For this review, take the finished solid that the model builds, in its own axes (mm). A direction names the side the tool comes from. Give positions to 0.01 mm unless a question says otherwise; leave off trailing zeros. Write each loop counter-clockwise with the first axis right and the second up, starting at its lowest first coordinate (ties: lowest second). Pieces come first, ordered by that corner, then holes. Notation, with made-up numbers: M -16,77.25 L 35,77.25 A22 ccw 35,104.25 Z; hole C 2.5,36.25 d7. An arc over 180 degrees is marked long. One line per item, written item: value. Start each with the question number.
Item 1: Consider section C-C, the plane z = 9.5. Write out the cut boundary in (x, y).
Item 2: Clearance check with flat-ended pins moving along their axes: pin 1 Ø4 at (x, z) = (11.5, -10.5) entering from +Y; pin 2 Ø1 at (x, z) = (-13, -1.5) entering from -Y; pin 3 Ø2 at (y, z) = (1.5, -8.5) entering from +X; pin 4 Ø8 at (y, z) = (4, 16.5) entering from +X. State where each tip first meets the part, or that it passes through.
Item 3: Consider section A-A, the plane x = 10.5. Write out the cut boundary in (y, z), and give its area (3 significant figures).
Item 4: Consider section B-B, the plane z = -3. Write out the cut boundary in (x, y).
Item 5: Consider section D-D, the plane x = 23. Write out the cut boundary in (y, z).
Item 6: To check wall thickness, follow probe 1 along Z at (x, y) = (-3, 1.5); probe 2 along X at (y, z) = (10.75, -2); probe 3 along Z at (x, y) = (-5, 11). State the ranges of each line that lie inside material, in increasing order.
Item 7: Mouldability with a two-part tool opening along Y and no side actions: class faces 1 (the face through (-15.5, 3, 25.7)), 2 (the face through (-4, 1, -1.328)) as released by +Y, released by -Y, zero draft, split by the parting line, or undercut.
Item 8: Tool access review of faces 3 (the face through (12, 1, -7.475)), 4 (the face through (21, 14, -4.468)), 5 (the face through (-13, 5, 2.366)), 6 (the face through (26, 13, 27)): name each direction out of +Z, -Z, +X, -X, +Y, -Y from which nothing blocks a thin tool from reaching the whole face with its end or side.
```python
from build123d import *

# Parameters (mm, degrees)
SKETCH1_W               = 36
SKETCH1_H               = 49
BOSS_EXTRUDE1_DEPTH     = 2
SKETCH2_W               = 36
SKETCH2_H               = 49
SKETCH2_W_2             = 32
SKETCH2_H_2             = 45
BOSS_EXTRUDE2_DEPTH     = 13
CUT_EXTRUDE1_DEPTH      = 5
CUT_EXTRUDE1_DEPTH_BACK = 48.529259103
SKETCH3_W               = 7.5
SKETCH3_H               = 2
SKETCH4_W               = 4.670437484
SKETCH4_H               = 3.853110924
CUT_EXTRUDE2_DEPTH      = 41.051989913
SKETCH10_W              = 2
SKETCH10_H              = 19
CUT_EXTRUDE6_DEPTH      = 3
SKETCH11_W              = 8
SKETCH11_H              = 7
CUT_EXTRUDE7_DEPTH      = 2
SKETCH12_W              = 5
SKETCH12_H              = 3
BOSS_EXTRUDE3_DEPTH     = 5
SKETCH13_W              = 5
SKETCH13_H              = 3
BOSS_EXTRUDE4_DEPTH     = 5
SKETCH14_R              = 0.775
CUT_EXTRUDE8_DEPTH      = 44.046736753
SKETCH15_R              = 1.275
CUT_EXTRUDE9_DEPTH      = 1
CUT_EXTRUDE10_START     = -1
SKETCH16_R              = 1.275
CUT_EXTRUDE10_DEPTH     = 1
FILLET2_R               = 10
SKETCH17_W              = 2
SKETCH17_H              = 4
CUT_EXTRUDE11_DEPTH     = 59.103279375
SKETCH18_W              = 2
SKETCH18_H              = 4
CUT_EXTRUDE12_DEPTH     = 53.763912582
SKETCH19_W              = 37.08283529
SKETCH19_H              = 2
CUT_EXTRUDE13_DEPTH     = 2
SKETCH20_W              = 37.08283529
SKETCH20_H              = 2
BOSS_EXTRUDE5_DEPTH     = 2
SKETCH21_W              = 2
SKETCH21_H              = 28
CUT_EXTRUDE14_DEPTH     = 2
SKETCH22_W              = 2
SKETCH22_H              = 28
BOSS_EXTRUDE6_DEPTH     = 2
SKETCH23_W              = 2
SKETCH23_H              = 34.1
CUT_EXTRUDE16_DEPTH     = 1.5
SKETCH24_W              = 2
SKETCH24_H              = 34.1
BOSS_EXTRUDE7_DEPTH     = 1.5


with BuildPart() as part:
    # Sketch1 → Boss-Extrude1 (new body)
    with BuildSketch(Plane(origin=(0, 0, 0), x_dir=(1, 0, 0), z_dir=(0, 1, 0))):
        with Locations((4.385964912, -5.131578947)):
            Rectangle(SKETCH1_W, SKETCH1_H)
    extrude(amount=BOSS_EXTRUDE1_DEPTH)

    # Sketch2 → Boss-Extrude2 (add)
    with BuildSketch(Plane(origin=(0, 2, 0), x_dir=(1, 0, 0), z_dir=(0, 1, 0))):
        with Locations((4.385964912, -5.131578947)):
            Rectangle(SKETCH2_W, SKETCH2_H)
        with Locations((4.385964912, -5.131578947)):
            Rectangle(SKETCH2_W_2, SKETCH2_H_2, mode=Mode.SUBTRACT)
    extrude(amount=BOSS_EXTRUDE2_DEPTH)

    # Sketch3 → Cut-Extrude1 (cut, two sides: drawn at the far end of the back side and taken through both)
    with BuildSketch(Plane.ZY.offset(-20.385964912).offset(-CUT_EXTRUDE1_DEPTH_BACK)):
        with Locations((-8.218421053, 14)):
            Rectangle(SKETCH3_W, SKETCH3_H)
    extrude(amount=CUT_EXTRUDE1_DEPTH + CUT_EXTRUDE1_DEPTH_BACK, mode=Mode.SUBTRACT)

    # Sketch4 → Cut-Extrude2 (cut, through all)
    with BuildSketch(Plane.XZ):
        with Locations((11.852478182, 20.598290589)):
            Rectangle(SKETCH4_W, SKETCH4_H)
        with Locations((-4.147521818, 20.598290589)):
            Rectangle(SKETCH4_W, SKETCH4_H)
        with Locations((11.852478182, 10.598290589)):
            Rectangle(SKETCH4_W, SKETCH4_H)
        with Locations((11.852478182, 0.598290589)):
            Rectangle(SKETCH4_W, SKETCH4_H)
        with Locations((11.852478182, -9.401709411)):
            Rectangle(SKETCH4_W, SKETCH4_H)
        with Locations((-4.147521818, 10.598290589)):
            Rectangle(SKETCH4_W, SKETCH4_H)
        with Locations((-4.147521818, 0.598290589)):
            Rectangle(SKETCH4_W, SKETCH4_H)
        with Locations((-4.147521818, -9.401709411)):
            Rectangle(SKETCH4_W, SKETCH4_H)
    extrude(amount=-CUT_EXTRUDE2_DEPTH, mode=Mode.SUBTRACT)

    # Sketch10 → Cut-Extrude6 (cut)
    with BuildSketch(Plane(origin=(0, 15, 0), x_dir=(1, 0, 0), z_dir=(0, 1, 0))):
        with Locations((-12.614035088, 7.868421053)):
            Rectangle(SKETCH10_W, SKETCH10_H)
    extrude(amount=-CUT_EXTRUDE6_DEPTH, mode=Mode.SUBTRACT)

    # Sketch11 → Cut-Extrude7 (cut)
    with BuildSketch(Plane.ZY.offset(13.614035088)):
        with Locations((-1.634350226, 5.5)):
            Rectangle(SKETCH11_W, SKETCH11_H)
    extrude(amount=-CUT_EXTRUDE7_DEPTH, mode=Mode.SUBTRACT)

    # Sketch12 → Boss-Extrude3 (add)
    with BuildSketch(Plane.ZY.offset(13.614035088)):
        with Locations((-16.868421053, 1.5)):
            Rectangle(SKETCH12_W, SKETCH12_H)
        with Locations((27.131578947, 13.5)):
            Rectangle(SKETCH12_W, SKETCH12_H)
        with Locations((27.131578947, 1.5)):
            Rectangle(SKETCH12_W, SKETCH12_H)
    extrude(amount=BOSS_EXTRUDE3_DEPTH)

    # Sketch13 → Boss-Extrude4 (add)
    with BuildSketch(Plane(origin=(22.385964912, 0, 0), x_dir=(0, 0, -1), z_dir=(1, 0, 0))):
        with Locations((16.868421053, 1.5)):
            Rectangle(SKETCH13_W, SKETCH13_H)
        with Locations((-27.131578947, 13.5)):
            Rectangle(SKETCH13_W, SKETCH13_H)
        with Locations((-27.131578947, 1.5)):
            Rectangle(SKETCH13_W, SKETCH13_H)
        with Locations((16.868421053, 13.5)):
            Rectangle(SKETCH13_W, SKETCH13_H)
    extrude(amount=BOSS_EXTRUDE4_DEPTH)

    # Sketch14 → Cut-Extrude8 (cut, through all)
    with BuildSketch(Plane.XZ):
        with Locations(Location((24.885964912, -16.868421053, 0), (0, 0, 270))):
            Circle(SKETCH14_R)
        with Locations(Location((-16.114035088, -16.868421053, 0), (0, 0, 270))):
            Circle(SKETCH14_R)
        with Locations(Location((-16.114035088, 27.131578947, 0), (0, 0, 270))):
            Circle(SKETCH14_R)
        with Locations(Location((24.885964912, 27.131578947, 0), (0, 0, 270))):
            Circle(SKETCH14_R)
    extrude(amount=-CUT_EXTRUDE8_DEPTH, mode=Mode.SUBTRACT)

    # Sketch15 → Cut-Extrude9 (cut)
    with BuildSketch(Plane(origin=(0, 3, 0), x_dir=(1, 0, 0), z_dir=(0, 1, 0))):
        with Locations(Location((24.885964912, 16.868421053, 0), (0, 0, 270))):
            Circle(SKETCH15_R)
        with Locations(Location((24.885964912, -27.131578947, 0), (0, 0, 270))):
            Circle(SKETCH15_R)
        with Locations(Location((-16.114035088, -27.131578947, 0), (0, 0, 270))):
            Circle(SKETCH15_R)
        with Locations(Location((-16.114035088, 16.868421053, 0), (0, 0, 270))):
            Circle(SKETCH15_R)
    extrude(amount=-CUT_EXTRUDE9_DEPTH, mode=Mode.SUBTRACT)

    # Sketch16 → Cut-Extrude10 (cut)
    with BuildSketch(Plane.XZ.offset(-12).offset(CUT_EXTRUDE10_START)):
        with Locations(Location((-16.114035088, 27.131578947, 0), (0, 0, 90))):
            Circle(SKETCH16_R)
        with Locations(Location((24.885964912, 27.131578947, 0), (0, 0, 90))):
            Circle(SKETCH16_R)
        with Locations(Location((24.885964912, -16.868421053, 0), (0, 0, 90))):
            Circle(SKETCH16_R)
    extrude(amount=CUT_EXTRUDE10_DEPTH, mode=Mode.SUBTRACT)

    # Fillet2
    # the kernel refuses this fillet: 10 mm, written as the material it adds along each edge
    with BuildSketch(Plane(origin=(-13.614035088, 0, -14.368421053), x_dir=(0, 0, 1), z_dir=(0, 1, 0)), Plane(origin=(22.385964912, 0, 24.631578947), x_dir=(0, 0, -1), z_dir=(0, 1, 0))) as fillet2_piece_1:
        with BuildLine():
            CenterArc((8.660254038, -10), FILLET2_R, 90, 60)
            Line((0, -5), (0, 0))
            Line((0, 0), (8.660254038, 0))
        make_face()
    extrude(amount=3)
    with BuildSketch(Plane(origin=(22.385964912, 0, -14.368421053), x_dir=(0, 0, 1), z_dir=(0, 1, 0)), Plane(origin=(-13.614035088, 0, 24.631578947), x_dir=(0, 0, -1), z_dir=(0, 1, 0))) as fillet2_piece_2:
        with BuildLine():
            CenterArc((8.660254038, 10), FILLET2_R, 210, 60)
            Line((0, 5), (0, 0))
            Line((0, 0), (8.660254038, 0))
        make_face()
    extrude(amount=3)

    # Sketch17 → Cut-Extrude11 (cut, through all)
    with BuildSketch(Plane.XY.offset(29.631578947)):
        with Locations((-3.340209091, 6.894489406)):
            Rectangle(SKETCH17_W, SKETCH17_H)
        with Locations((5.343190897, 6.894489406)):
            Rectangle(SKETCH17_W, SKETCH17_H)
        with Locations((13.309543319, 6.894489406)):
            Rectangle(SKETCH17_W, SKETCH17_H)
    extrude(amount=-CUT_EXTRUDE11_DEPTH, mode=Mode.SUBTRACT)

    # Sketch18 → Cut-Extrude12 (cut, through all)
    with BuildSketch(Plane.ZY.offset(13.614035088)):
        with Locations((11.893757697, 6.4242408)):
            Rectangle(SKETCH18_W, SKETCH18_H)
        with Locations((19.784308777, 6.4242408)):
            Rectangle(SKETCH18_W, SKETCH18_H)
    extrude(amount=-CUT_EXTRUDE12_DEPTH, mode=Mode.SUBTRACT)

    # Sketch19 → Cut-Extrude13 (cut)
    with BuildSketch(Plane(origin=(0, 15, 0), x_dir=(1, 0, 0), z_dir=(0, 1, 0))):
        with Locations((4.927382557, 18.368421053)):
            Rectangle(SKETCH19_W, SKETCH19_H)
    extrude(amount=-CUT_EXTRUDE13_DEPTH, mode=Mode.SUBTRACT)

    # Sketch20 → Boss-Extrude5 (add)
    with BuildSketch(Plane(origin=(0, 13, 0), x_dir=(1, 0, 0), z_dir=(0, 1, 0))):
        with Locations((4.927382557, 18.368421053)):
            Rectangle(SKETCH20_W, SKETCH20_H)
    extrude(amount=BOSS_EXTRUDE5_DEPTH)

    # Sketch21 → Cut-Extrude14 (cut)
    with BuildSketch(Plane(origin=(0, 15, 0), x_dir=(1, 0, 0), z_dir=(0, 1, 0))):
        with Locations((-12.614035088, -15.631578947)):
            Rectangle(SKETCH21_W, SKETCH21_H)
    extrude(amount=-CUT_EXTRUDE14_DEPTH, mode=Mode.SUBTRACT)

    # Sketch22 → Boss-Extrude6 (add)
    with BuildSketch(Plane(origin=(0, 13, 0), x_dir=(1, 0, 0), z_dir=(0, 1, 0))):
        with Locations((-12.614035088, -15.631578947)):
            Rectangle(SKETCH22_W, SKETCH22_H)
    extrude(amount=BOSS_EXTRUDE6_DEPTH)

    # Sketch23 → Cut-Extrude16 (cut)
    with BuildSketch(Plane(origin=(0, 15, 0), x_dir=(1, 0, 0), z_dir=(0, 1, 0))):
        with Locations((21.385964912, -12.581578947)):
            Rectangle(SKETCH23_W, SKETCH23_H)
    extrude(amount=-CUT_EXTRUDE16_DEPTH, mode=Mode.SUBTRACT)

    # Sketch24 → Boss-Extrude7 (add)
    with BuildSketch(Plane(origin=(0, 13.5, 0), x_dir=(1, 0, 0), z_dir=(0, 1, 0))):
        with Locations((21.385964912, -12.581578947)):
            Rectangle(SKETCH24_W, SKETCH24_H)
    extrude(amount=BOSS_EXTRUDE7_DEPTH)


solid = part.part
```
Model answer:
1. outline: M -13.61,0 L -6.48,0 L -6.48,2 L -11.61,2 L -11.61,15 L -13.61,15 Z; M -1.81,0 L 9.52,0 L 9.52,2 L -1.81,2 Z; M 14.19,0 L 22.39,0 L 22.39,15 L 20.39,15 L 20.39,2 L 14.19,2 Z
2. pin 1: stops at y = 2
2. pin 2: stops at y = 0
2. pin 3: stops at x = 23.13
2. pin 4: stops at x = 23.41
3. outline: M 0,-19.37 L 15,-19.37 L 15,-17.37 L 2,-17.37 L 2,-11.33 L 0,-11.33 Z; M 0,-7.48 L 2,-7.48 L 2,-1.33 L 0,-1.33 Z; M 0,2.52 L 2,2.52 L 2,8.67 L 0,8.67 Z; M 0,12.52 L 2,12.52 L 2,18.67 L 0,18.67 Z; M 0,22.52 L 2,22.52 L 2,27.63 L 15,27.63 L 15,29.63 L 0,29.63 Z
3. area: 119 mm2
4. outline: M -13.61,0 L 22.39,0 L 22.39,15 L 20.39,15 L 20.39,2 L -13.61,2 Z; M -13.61,9 L -11.61,9 L -11.61,12 L -13.61,12 Z
5. outline: M 0,-19.37 L 3,-19.37 L 3,-9.16 L 0,-9.16 Z; M 0,19.42 L 3,19.42 L 3,29.63 L 0,29.63 Z; M 12,-19.37 L 15,-19.37 L 15,-14.37 L 12,-14.37 Z; M 12,24.63 L 15,24.63 L 15,29.63 L 12,29.63 Z
6. probe 1: z = -19.37 to -11.33, -7.48 to -1.33, 2.52 to 8.67, 12.52 to 18.67, 22.52 to 29.63
6. probe 2: x = -13.61 to -11.61, 20.39 to 22.39
6. probe 3: z = -19.37 to -17.37, 27.63 to 29.63
7. face 1: undercut
7. face 2: zero draft
8. face 3: +Y, -Y
8. face 4: +X, -X, +Y
8. face 5: -X
8. face 6: none
